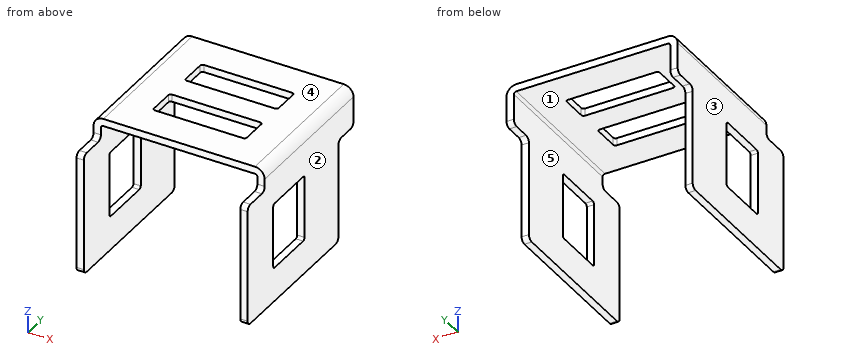
```python
from build123d import *

# Parameters (mm, degrees)
SKETCH1_W           = 37.2
SKETCH1_H           = 29.5
BOSS_EXTRUDE1_DEPTH = 1.5
SKETCH2_W           = 4.5
SKETCH2_H           = 6
CUT_EXTRUDE1_DEPTH  = 2.5
SKETCH3_W           = 1.5
SKETCH3_H           = 31.2
BOSS_EXTRUDE2_DEPTH = 33.5
SKETCH4_W           = 1.5
SKETCH4_H           = 31.2
BOSS_EXTRUDE3_DEPTH = 28
SKETCH5_W           = 1.5
SKETCH5_H           = 25
BOSS_EXTRUDE4_DEPTH = 6
CUT_EXTRUDE2_REACH  = 37
SKETCH6_W           = 21.3
SKETCH6_H           = 5.3
SKETCH7_W           = 21.3
SKETCH7_H           = 5.3
CUT_EXTRUDE3_DEPTH  = 36
FILLET1_R           = 0.5
FILLET2_R           = 2
SKETCH8_W           = 19
SKETCH8_H           = 6
CUT_EXTRUDE4_DEPTH  = 1.5
FILLET3_R           = 0.5
SKETCH9_W           = 13.5
SKETCH9_H           = 11
CUT_EXTRUDE5_DEPTH  = 35
FILLET4_R           = 0.5
FILLET5_R           = 1


with BuildPart() as part:
    # Sketch1 → Boss-Extrude1 (new body)
    with BuildSketch(Plane(origin=(16, 0, 0), x_dir=(0, -1, 0), z_dir=(-1, 0, 0))):
        with Locations((46.1, 3.75)):
            Rectangle(SKETCH1_W, SKETCH1_H)
    extrude(amount=-BOSS_EXTRUDE1_DEPTH)

    # Sketch2 → Cut-Extrude1 (cut, through all)
    with BuildSketch(Plane(origin=(17.5, 0, 0), x_dir=(0, 0, -1), z_dir=(1, 0, 0))):
        with Locations((-16.25, -61.7)):
            Rectangle(SKETCH2_W, SKETCH2_H)
    extrude(amount=-CUT_EXTRUDE1_DEPTH, mode=Mode.SUBTRACT)

    # Sketch3 → Boss-Extrude2 (add)
    with BuildSketch(Plane.ZY.offset(-16)):
        with Locations((17.75, -43.1)):
            Rectangle(SKETCH3_W, SKETCH3_H)
    extrude(amount=BOSS_EXTRUDE2_DEPTH)

    # Sketch4 → Boss-Extrude3 (add)
    with BuildSketch(Plane(origin=(0, 0, 17), x_dir=(-1, 0, 0), z_dir=(0, 0, -1))):
        with Locations((16.75, -43.1)):
            Rectangle(SKETCH4_W, SKETCH4_H)
    extrude(amount=BOSS_EXTRUDE3_DEPTH)

    # Sketch5 → Boss-Extrude4 (add)
    with BuildSketch(Plane.XZ.offset(58.7)):
        with Locations((-16.75, 1.5)):
            Rectangle(SKETCH5_W, SKETCH5_H)
    extrude(amount=BOSS_EXTRUDE4_DEPTH)

    # Sketch6 → Cut-Extrude2 (cut, up to next)
    with BuildSketch(Plane(origin=(17.5, 0, 0), x_dir=(0, 0, -1), z_dir=(1, 0, 0)), mode=Mode.PRIVATE) as cut_extrude2_sk1:
        with Locations((0.35, -30.15)):
            Rectangle(SKETCH6_W, SKETCH6_H)
    cut_extrude2_tool1 = extrude(cut_extrude2_sk1.sketch, amount=-CUT_EXTRUDE2_REACH, mode=Mode.PRIVATE) & part.part
    add(cut_extrude2_tool1.solids().sort_by_distance((17.5, -30.15, -0.35))[0], mode=Mode.SUBTRACT)

    # Sketch7 → Cut-Extrude3 (cut, through all)
    with BuildSketch(Plane.ZY.offset(17.5)):
        with Locations((-0.35, -30.15)):
            Rectangle(SKETCH7_W, SKETCH7_H)
    extrude(amount=-CUT_EXTRUDE3_DEPTH, mode=Mode.SUBTRACT)

    # Fillet1
    fillet1_edges = [part.edges().sort_by_distance(p)[0] for p in [
        (16, -43.1, 17),
        (-16, -43.1, 17),
    ]]
    fillet(fillet1_edges, radius=FILLET1_R)

    # Fillet2
    fillet2_edges = [part.edges().sort_by_distance(p)[0] for p in [
        (17.5, -43.1, 18.5),
        (-17.5, -43.1, 18.5),
    ]]
    fillet(fillet2_edges, radius=FILLET2_R)

    # Sketch8 → Cut-Extrude4 (cut)
    with BuildSketch(Plane.XY.offset(18.5)):
        with Locations((0, -37.5)):
            Rectangle(SKETCH8_W, SKETCH8_H)
        with Locations((0, -48.7)):
            Rectangle(SKETCH8_W, SKETCH8_H)
    extrude(amount=-CUT_EXTRUDE4_DEPTH, mode=Mode.SUBTRACT)

    # Fillet3
    fillet3_edges = [part.edges().sort_by_distance(p)[0] for p in [
        (9.5, -51.7, 17.75),
        (-9.5, -51.7, 17.75),
        (-9.5, -45.7, 17.75),
        (9.5, -45.7, 17.75),
        (-9.5, -40.5, 17.75),
        (-9.5, -34.5, 17.75),
        (9.5, -34.5, 17.75),
        (9.5, -40.5, 17.75),
    ]]
    fillet(fillet3_edges, radius=FILLET3_R)

    # Sketch9 → Cut-Extrude5 (cut)
    with BuildSketch(Plane(origin=(17.5, 0, 0), x_dir=(0, 0, -1), z_dir=(1, 0, 0))):
        with Locations((-2.75, -50.2)):
            Rectangle(SKETCH9_W, SKETCH9_H)
    extrude(amount=-CUT_EXTRUDE5_DEPTH, mode=Mode.SUBTRACT)

    # Fillet4
    fillet4_edges = [part.edges().sort_by_distance(p)[0] for p in [
        (-16.75, -55.7, 9.5),
        (-16.75, -44.7, 9.5),
        (-16.75, -44.7, -4),
        (-16.75, -55.7, -4),
        (16.75, -55.7, 9.5),
        (16.75, -44.7, 9.5),
        (16.75, -44.7, -4),
        (16.75, -55.7, -4),
    ]]
    fillet(fillet4_edges, radius=FILLET4_R)

    # Fillet5
    fillet5_edges = [part.edges().sort_by_distance(p)[0] for p in [
        (16.75, -58.7, 14),
        (16.75, -64.7, 14),
        (-16.75, -58.7, 14),
        (-16.75, -64.7, -11),
        (-16.75, -64.7, 14),
        (16.75, -32.8, -11),
        (16.75, -32.8, 10.3),
        (16.75, -27.5, 10.3),
        (16.75, -64.7, -11),
        (-16.75, -27.5, 10.3),
        (-16.75, -32.8, -11),
        (-16.75, -32.8, 10.3),
    ]]
    fillet(fillet5_edges, radius=FILLET5_R)


solid = part.part
```
Model file for the job. Use its own axes, mm. Face numbers are marked on the shaded views. A direction names the side the tool comes from. Give positions to 0.01 mm unless a question says otherwise; leave off trailing zeros. Loops run counter-clockwise (first coordinate to the right, second up) from the corner with the lowest first, then second, coordinate; pieces in that order, holes last. Notation, with made-up numbers: (64, 61.25) - (121, 61.25) arc R18 cw to (121, 84.25) - close; hole circle Ø10 at (10.25, 15). An arc over 180 degrees is marked (long way). One line per item, written item: value. Start each with the question number.
1. Pin check, flat tips, straight feed: pin 1 (0.8 mm diameter, centred on y = -38, z = 17.5, fed in from -X); pin 2 (1.2 mm diameter, centred on x = -16.5, y = -30, fed in from -Z); pin 3 (1.6 mm diameter, centred on x = -16.5, y = -62, fed in from +Z). Stop position of each tip, or through.
2. Pull direction X, two halves, no side cores. Call the marked faces 1, 2 and 3: pulls with the +X half, pulls with the -X half, needs draft (parallel to the pull), parting line crosses it, or undercut.
3. Slice it at D-D (y = -48). List the corners of the cut face in (x, z).
4. Which spindle directions (+Z, -Z, +X, -X, +Y, -Y) get a long thin tool onto all of the face, cutting with end or side? Do the marked faces 4 and 5. Say none if no direction does.
5. Slice it at C-C (y = -37.5). List the corners of the cut face in (x, z), plus the area to 3 significant figures.
6. Slice it at B-B (x = -4). List the corners of the cut face in (y, z), plus the area to 3 significant figures.
7. Slice it at A-A (z = 4.5). List the corners of the cut face in (x, y).
8. Probe L1, parallel to X at y = -39, z = -4.25; L2, parallel to Z at x = 1, y = -54. List the from-to ranges inside material, lowest first. Write a range as from..to.
Solution:
1. pin 1: stops at x = -17.41
1. pin 2: stops at z = 10.3
1. pin 3: stops at z = 14
2. face 1: undercut
2. face 2: pulls with the +X half
2. face 3: pulls with the -X half
3. outline: (-17.5, -11) - (-16, -11) - (-16, -4) - (-17.5, -4) - close; (-17.5, 9.5) - (-16, 9.5) - (-16, 16.5) arc R0.5 cw to (-15.5, 17) - (-9.5, 17) - (-9.5, 18.5) - (-15.5, 18.5) arc R2 ccw to (-17.5, 16.5) - close; (9.5, 17) - (15.5, 17) arc R0.5 cw to (16, 16.5) - (16, 9.5) - (17.5, 9.5) - (17.5, 16.5) arc R2 ccw to (15.5, 18.5) - (9.5, 18.5) - close; (16, -11) - (17.5, -11) - (17.5, -4) - (16, -4) - close
4. face 4: +Z, +X, -X, +Y, -Y
4. face 5: -Z, +Y, -Y
5. outline: (-17.5, -11) - (-16, -11) - (-16, 16.5) arc R0.5 cw to (-15.5, 17) - (-9.5, 17) - (-9.5, 18.5) - (-15.5, 18.5) arc R2 ccw to (-17.5, 16.5) - close; (9.5, 17) - (15.5, 17) arc R0.5 cw to (16, 16.5) - (16, -11) - (17.5, -11) - (17.5, 16.5) arc R2 ccw to (15.5, 18.5) - (9.5, 18.5) - close
5. area: 106 mm^2
6. outline: (-58.7, 17) - (-51.7, 17) - (-51.7, 18.5) - (-58.7, 18.5) - close; (-45.7, 17) - (-40.5, 17) - (-40.5, 18.5) - (-45.7, 18.5) - close; (-34.5, 17) - (-27.5, 17) - (-27.5, 18.5) - (-34.5, 18.5) - close
6. area: 28.8 mm^2
7. outline: (-17.5, -64.7) - (-16, -64.7) - (-16, -55.7) - (-17.5, -55.7) - close; (-17.5, -44.7) - (-16, -44.7) - (-16, -32.8) - (-17.5, -32.8) - close; (16, -64.7) - (17.5, -64.7) - (17.5, -55.7) - (16, -55.7) - close; (16, -44.7) - (17.5, -44.7) - (17.5, -32.8) - (16, -32.8) - close
8. L1: x = -17.5..-16, 16..17.5
8. L2: z = 17..18.5
